Part print with two shaded views. Sizes in mm from the minimum x, y, z corner. Round coordinates to 2 decimals unless told otherwise and drop trailing zeros. Loops run counter-clockwise (first coordinate to the right, second up) from the corner with the lowest first, then second, coordinate; pieces in that order, holes last.
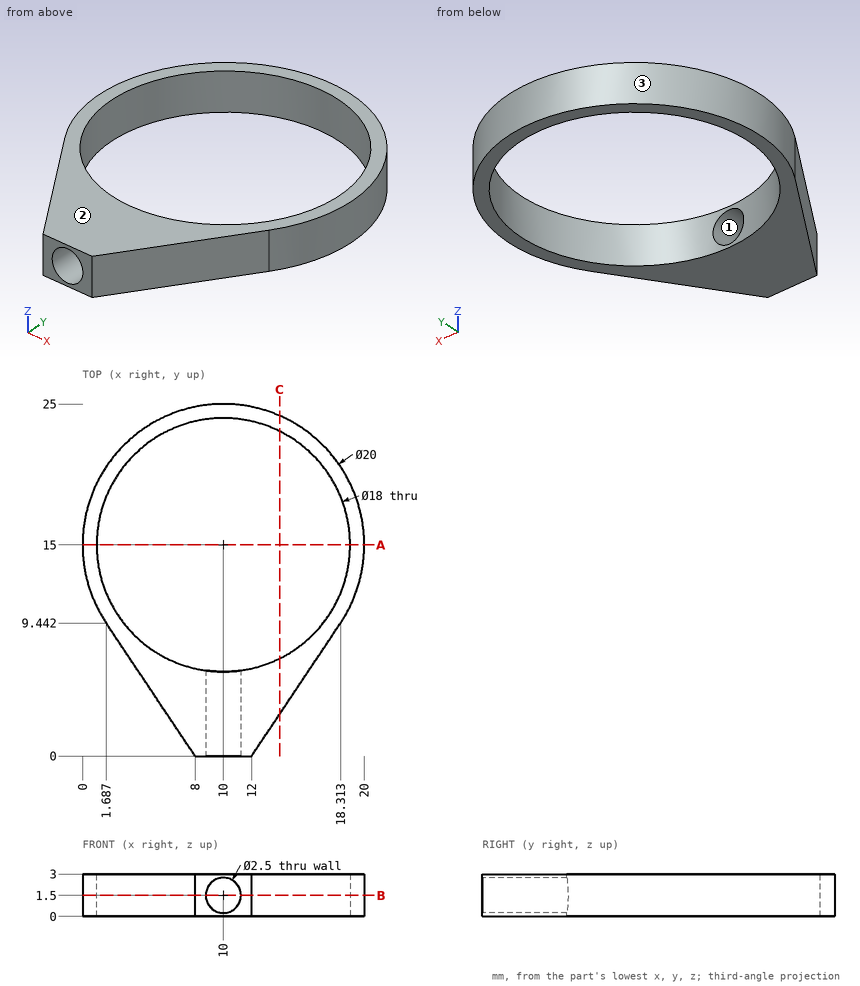
Item 1: Cut at C-C (x = 14). List the corners of the cut face in (y, z) (1 decimal).
Verdict:
outline: (3, 0) - (6.9, 0) - (6.9, 3) - (3, 3) - close; (23.1, 0) - (24.2, 0) - (24.2, 3) - (23.1, 3) - close
Item 2: Flat gauge pins, fed straight in: P1, Ø1, axis at x = 4, z = 1, coming from the -Y side (1 decimal); P2, Ø1.5, axis at y = 14, z = 1, coming from the -X side; P3, Ø1, axis at y = 7, z = 2, coming from the +X side (1 decimal). Where does each tip first touch, or does it go through?
Verdict:
P1: stops at y = 5.2
P2: stops at x = 0
P3: stops at x = 17
Item 3: Cut at A-A (y = 15). List the corners of the cut face in (x, z).
Verdict:
outline: (0, 0) - (1, 0) - (1, 3) - (0, 3) - close; (19, 0) - (20, 0) - (20, 3) - (19, 3) - close
Item 4: Wall check: L1, parallel to Y at x = 10.25, z = 0.2; L2, parallel to Y at x = 10.25, z = 2.25; L3, parallel to X at y = 22.75, z = 2.3 (1 decimal). Give the ranges that are in metal, low to high.
Verdict:
L1: y = 0 to 6, 24 to 25
L2: y = 24 to 25
L3: x = 3.7 to 5.4, 14.6 to 16.3
Item 5: Cut at B-B (z = 1.5). List the corners of the cut face in (x, y).
Verdict:
outline: (1.69, 9.44) - (8, 0) - (8.75, 0) - (8.75, 6.09) arc R9 cw (long way) to (11.25, 6.09) - (11.25, 0) - (12, 0) - (18.31, 9.44) arc R10 ccw (long way) to start
Item 6: Mould opens along X. For the marked faces 1, 2 and 3 say: released by +X, released by -X, zero draft, split by the parting line, or undercut.
Verdict:
face 1: undercut
face 2: zero draft
face 3: split by the parting line
